Here's how the part is built. I have some questions about the finished solid (model axes, mm). Round coordinates to 2 decimals unless told otherwise and drop trailing zeros. Write each loop counter-clockwise with the first axis right and the second up, starting at its lowest first coordinate (ties: lowest second). Pieces come first, ordered by that corner, then holes. Notation, with made-up numbers: (68.25, 58) -> (120.25, 58) arc R27 cw to (120.25, 83) -> close; hole circle Ø6 at (74, 17). An arc over 180 degrees is marked (long way). Answer as CSV lines item,"result".
from build123d import *

# Parameters (mm, degrees)
SKETCH_1_W     = 27
SKETCH_1_H     = 3
CHAMFER_1_SIZE = 0.5


with BuildPart() as part:
    # 草图1 → 旋转1 (revolve)
    with BuildSketch(Plane(origin=(-4266.423458032, -24.943356191, -7335.56447096), x_dir=(-1, 0, 0), z_dir=(0, -0.999994681, 0.00326158))):
        with Locations((-4216.678380328, -7394.483238222)):
            Rectangle(SKETCH_1_W, SKETCH_1_H)
    revolve(axis=Axis((-153.375983394, -0.762059862, 78.379332546), (1, 0, 0)))

    # 倒角1
    chamfer_1_edges = [part.edges().sort_by_distance(p)[0] for p in [
        (-63.245077704, -0.693566691, 99.379220848),
        (-36.245077704, -0.693566691, 99.379220848),
        (-36.245077704, -0.70335143, 96.379236805),
        (-63.245077704, -0.70335143, 96.379236805),
    ]]
    chamfer(chamfer_1_edges, length=CHAMFER_1_SIZE)


solid = part.part
Item 1: Will these pins go through, and if not, where does the flat tip stop? pin 1 (1 mm diameter, centred on x = -43, y = 1.5, fed in from +Z); pin 2 (2 mm diameter, centred on y = 15.5, z = 91.5, fed in from -X); pin 3 (4 mm diameter, centred on x = -44.5, z = 72, fed in from -Y); pin 4 (2 mm diameter, centred on x = -49.5, z = 72, fed in from +Y).
Results found:
pin 1,"stops at z = 99.31"
pin 2,"stops at x = -63.25"
pin 3,"stops at y = -21.3"
pin 4,"stops at y = 19.54"
Item 2: Suppose I cut it at A-A, the plane x = -58.5. List the corners of the cut face in (y, z) for me.
Results found:
outline,"circle Ø42 at (-0.76, 78.38); hole circle Ø36 at (-0.76, 78.38)"
Item 3: I need wall thicknesses on L1, parallel to Y at x = -57.25, z = 78; L2, parallel to Z at x = -55.25, y = -0.5; L3, parallel to Y at x = -45, z = 62. Which ranges of each line are inside material? Lowest first, please.
Results found:
L1,"y = -21.76 to -18.76, 17.23 to 20.23"
L2,"z = 57.38 to 60.38, 96.38 to 99.38"
L3,"y = -13.9 to -8.23, 6.7 to 12.38"
Item 4: If we mould it in two halves opening along Z, with no side actions, what happens to faces 1 (the flat face through (-63.245, 18, 75)), 2 (the cylindrical face through (-49.93, 0.09, 96.36)), 3 (the cylindrical face through (-49.927, -13.486, 95.086))? For each: pulls with the +Z half, pulls with the -Z half, needs draft (parallel to the pull), parting line crosses it, or undercut.
Results found:
face 1,"needs draft"
face 2,"undercut"
face 3,"parting line crosses it"
